```python
from build123d import *

# Parameters (mm, degrees)
SKETCH1_R           = 2
BOSS_EXTRUDE1_DEPTH = 2
SKETCH2_R           = 1.25
BOSS_EXTRUDE2_DEPTH = 10
FILLET1_R           = 0.3
CUT_EXTRUDE1_DEPTH  = 1.5


with BuildPart() as part:
    # Sketch1 → Boss-Extrude1 (new body)
    with BuildSketch(Plane(origin=(0, 0, 0), x_dir=(1, 0, 0), z_dir=(0, 1, 0))):
        Circle(SKETCH1_R)
    extrude(amount=BOSS_EXTRUDE1_DEPTH)

    # Sketch2 → Boss-Extrude2 (add)
    with BuildSketch(Plane.XZ):
        Circle(SKETCH2_R)
    extrude(amount=BOSS_EXTRUDE2_DEPTH)

    # Fillet1
    fillet1_edges = [part.edges().sort_by_distance(p)[0] for p in [
        (-2, 2, 0),
    ]]
    fillet(fillet1_edges, radius=FILLET1_R)

    # Sketch4 → Cut-Extrude1 (cut)
    with BuildSketch(Plane(origin=(0, 2, 0), x_dir=(1, 0, 0), z_dir=(0, 1, 0))):
        Polygon((1.299038106, 0), (0.649519053, 1.125), (-0.649519053, 1.125), (-1.299038106, 0), (-0.649519053, -1.125), (0.649519053, -1.125), align=None)
    extrude(amount=-CUT_EXTRUDE1_DEPTH, mode=Mode.SUBTRACT)


solid = part.part
```
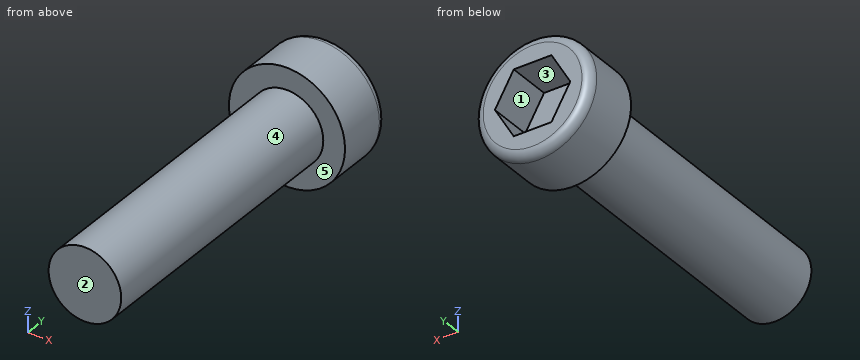
Check sheet for the modelled part. Datum: model origin and axes. Units: mm. Face numbers are marked on the shaded views. A direction names the side the tool comes from. Coordinates: 2 decimals unless noted, no trailing zeros. Write each loop counter-clockwise with the first axis right and the second up, starting at its lowest first coordinate (ties: lowest second). Pieces come first, ordered by that corner, then holes. Notation, with made-up numbers: M 68.5,74.25 L 98.5,74.25 A20 ccw 98.5,89.25 Z; hole C -38,75.25 d5. An arc over 180 degrees is marked long. Use one line per item in the form item = value.
Item 1: Release check for a two-part mould opening along X. For the marked faces 3, 4 and 5 record: pulls with the +X half, pulls with the -X half, needs draft (parallel to the pull), parting line crosses it, or undercut.
Answer below:
face_3 = undercut
face_4 = parting line crosses it
face_5 = needs draft
Item 2: Sectioned sample at A-A, the plane y = 1.25. Record the cut outline in (x, z) (3 decimals).
Answer below:
outline = C 0,0 d4; hole M -1.299,0 L -0.65,-1.125 L 0.65,-1.125 L 1.299,0 L 0.65,1.125 L -0.65,1.125 Z
Item 3: Sectioned sample at C-C, the plane y = -6.75. Record the cut outline in (x, z), and give its area (3 significant figures).
Answer below:
outline = C 0,0 d2.5
area = 4.91 mm^2
Item 4: Set-up check for the marked faces 1 and 2: record each of +Z, -Z, +X, -X, +Y, -Y from which the full face is reachable in a straight line by a thin tool's end or side.
Answer below:
face_1 = +Y
face_2 = +Z, -Z, +X, -X, -Y
Item 5: Sectioned sample at B-B, the plane x = 0. Record the cut outline in (y, z) (3 decimals).
Answer below:
outline = M -10,-1.25 L 0,-1.25 L 0,-2 L 1.7,-2 A0.3 ccw 2,-1.7 L 2,-1.125 L 0.5,-1.125 L 0.5,1.125 L 2,1.125 L 2,1.7 A0.3 ccw 1.7,2 L 0,2 L 0,1.25 L -10,1.25 Z
Item 6: Material ranges on L1, parallel to Y at x = 0.1, z = 0.4; L2, parallel to Z at x = 0.05, y = -5.5; L3, parallel to Y at x = -1.55, z = 0.8, recorded low to high. Write a range as from..to.
Answer below:
L1 = -10..0.5
L2 = -1.25..1.25
L3 = 0..2
Item 7: Gauge pin test, flat ends, axial feed: pin 1 Ø1.5 at (y, z) = (0.5, -1.5) entering from -X; pin 2 Ø1.5 at (y, z) = (-5, -0.5) entering from +X; pin 3 Ø0.6 at (x, y) = (-0.5, 1.5) entering from -Z. Record the tip position at first contact, or that the pin passes through.
Answer below:
pin_1 = -1.85
pin_2 = 1.25
pin_3 = -1.99
